The listing builds one solid part. Answer for the finished solid, in the listing's coordinates (mm). Give positions to 0.01 mm unless a question says otherwise; leave off trailing zeros. Write each loop counter-clockwise with the first axis right and the second up, starting at its lowest first coordinate (ties: lowest second). Pieces come first, ordered by that corner, then holes. Notation, with made-up numbers: M 71,22.25 L 115,22.25 A4 cw 115,27.25 Z; hole C 45.25,30 d9. An arc over 180 degrees is marked long. Answer as a JSON object with one key per item and string values.
```python
from build123d import *

# Parameters (mm, degrees)
SKETCH1_R           = 8
SKETCH1_R_2         = 7
BOSS_EXTRUDE1_DEPTH = 305
SKETCH2_R           = 1.05
CUT_EXTRUDE2_DEPTH  = 20


with BuildPart() as part:
    # Sketch1 → Boss-Extrude1 (new body)
    with BuildSketch(Plane.XY):
        Circle(SKETCH1_R)
        Circle(SKETCH1_R_2, mode=Mode.SUBTRACT)
    extrude(amount=BOSS_EXTRUDE1_DEPTH)

    # Sketch2 → Cut-Extrude2 (cut)
    with BuildSketch(Plane.XZ.offset(10)):
        with Locations(Location((0, 2.5, 0), (0, 0, 270))):
            Circle(SKETCH2_R)
        with Locations(Location((0, 56.5, 0), (0, 0, 270))):
            Circle(SKETCH2_R)
        with Locations(Location((0, 255.1, 0), (0, 0, 270))):
            Circle(SKETCH2_R)
        with Locations(Location((0, 303, 0), (0, 0, 270))):
            Circle(SKETCH2_R)
    extrude(amount=-CUT_EXTRUDE2_DEPTH, mode=Mode.SUBTRACT)


solid = part.part
```
1. Consider line 1 along Z through (x, y) = (0, 7.6); line 2 along Y through (x, z) = (0, 241.5); line 3 along X through (y, z) = (-5.75, 43.5). Determine where each line is inside the solid, lowest interval first.
Verdict:
{"line 1": "z = 0 to 1.45, 3.55 to 55.45, 57.55 to 254.05, 256.15 to 301.95, 304.05 to 305", "line 2": "y = -8 to -7, 7 to 8", "line 3": "x = -5.56 to -3.99, 3.99 to 5.56"}
2. A cutting plane is placed at B-B, the plane x = 4. Give the vertices of the cut face in (y, z).
Verdict:
{"outline": "M -6.93,0 L -5.74,0 L -5.74,305 L -6.93,305 Z; M 5.74,0 L 6.93,0 L 6.93,305 L 5.74,305 Z"}
3. A cutting plane is placed at C-C, the plane z = 205. Give the vertices of the cut face in (x, y).
Verdict:
{"outline": "C 0,0 d16; hole C 0,0 d14"}
4. A cutting plane is placed at A-A, the plane y = 0. Give the vertices of the cut face in (x, z).
Verdict:
{"outline": "M -8,0 L -7,0 L -7,305 L -8,305 Z; M 7,0 L 8,0 L 8,305 L 7,305 Z"}
5. Flat-ended cylindrical pins translate along their axes: pin 1 (2.5 mm diameter, centred on x = 0, z = 2.5, fed in from +Y); pin 2 (1.9 mm diameter, centred on x = 0, z = 255.1, fed in from -Y); pin 3 (4 mm diameter, centred on y = -4, z = 142.5, fed in from -X); pin 4 (1 mm diameter, centred on y = 5.5, z = 166, fed in from +X) (3 decimals). Find the tip coordinate at first contact, or state that the pin passes through.
Verdict:
{"pin 1": "stops at y = 8", "pin 2": "passes through", "pin 3": "stops at x = -7.75", "pin 4": "stops at x = 6.245"}
